Geometry: final body of the model. Coordinates: model frame, mm. A direction names the side the tool comes from. Give positions to 0.01 mm unless a question says otherwise; leave off trailing zeros. Write each loop counter-clockwise with the first axis right and the second up, starting at its lowest first coordinate (ties: lowest second). Pieces come first, ordered by that corner, then holes.
from build123d import *

# Parameters (mm, degrees)
F1_DEPTH = 5.5
F2_R     = 4
F3_DEPTH = 40
F4_SIZE  = 0.4


with BuildPart() as f1:
    # F0 (on Top) → F1 (new body)
    with BuildSketch(Plane.XY):
        Polygon((6.5, 3.752777), (0, 7.505553), (-6.5, 3.752777), (-6.5, -3.752777), (0, -7.505553), (6.5, -3.752777), align=None)
    extrude(amount=F1_DEPTH)

    # F2 (on face) → F3 (join)
    with BuildSketch(Plane.XY.offset(5.5)):
        Circle(F2_R)
    extrude(amount=F3_DEPTH)

    # F4
    f4_edges = [f1.edges().sort_by_distance(p)[0] for p in [
        (-4, 0, 45.5),
    ]]
    chamfer(f4_edges, length=F4_SIZE)

    # F5 (on Front) → F6 (revolve, cut)
    with BuildSketch(Plane.XZ):
        Polygon((-11.5, 1), (-11.5, 0), (-6.5, 0), align=None)
    revolve(axis=Axis((0, 0, 5.5), (0, 0, -1)), mode=Mode.SUBTRACT)


solid = f1.part
Q1. Ray query, line 1 along Z through (x, y) = (-2, 3.5); line 2 along Y through (x, z) = (-0.25, 43); line 3 along Z through (x, y) = (-2, -3). Return the intervals inside material, ascending.
Filled sheet:
line 1: z = 0 to 5.5
line 2: y = -3.99 to 3.99
line 3: z = 0 to 45.49
Q2. Section A-A on z = 29. Output: boundary loops of the cut face in (x, y).
Filled sheet:
outline: circle Ø8 at (0, 0)
Q3. Access query for faces 1 (the cylindrical face through (-0.867, -3.905, 25.023)), 2 (the flat face through (0, 0, 0)). Directions: +Z, -Z, +X, -X, +Y, -Y. A direction counts if a zero-diameter tool reaches every point of the face in a straight line with its end or side. Return the directions, or none.
Filled sheet:
face 1: +Z
face 2: -Z, +X, -X, +Y, -Y
Q4. Pin query (flat end, axial travel): P1, Ø1, axis at y = 5.5, z = 30, coming from the +X side; P2, Ø5, axis at y = -4, z = 35, coming from the +X side; P3, Ø8, axis at y = 2, z = 38.5, coming from the -X side; P4, Ø4, axis at y = -2, z = 41, coming from the +X side. Return the tip coordinate at first contact, or that it passes through.
Filled sheet:
P1: passes through
P2: stops at x = 3.71
P3: stops at x = -4
P4: stops at x = 4
